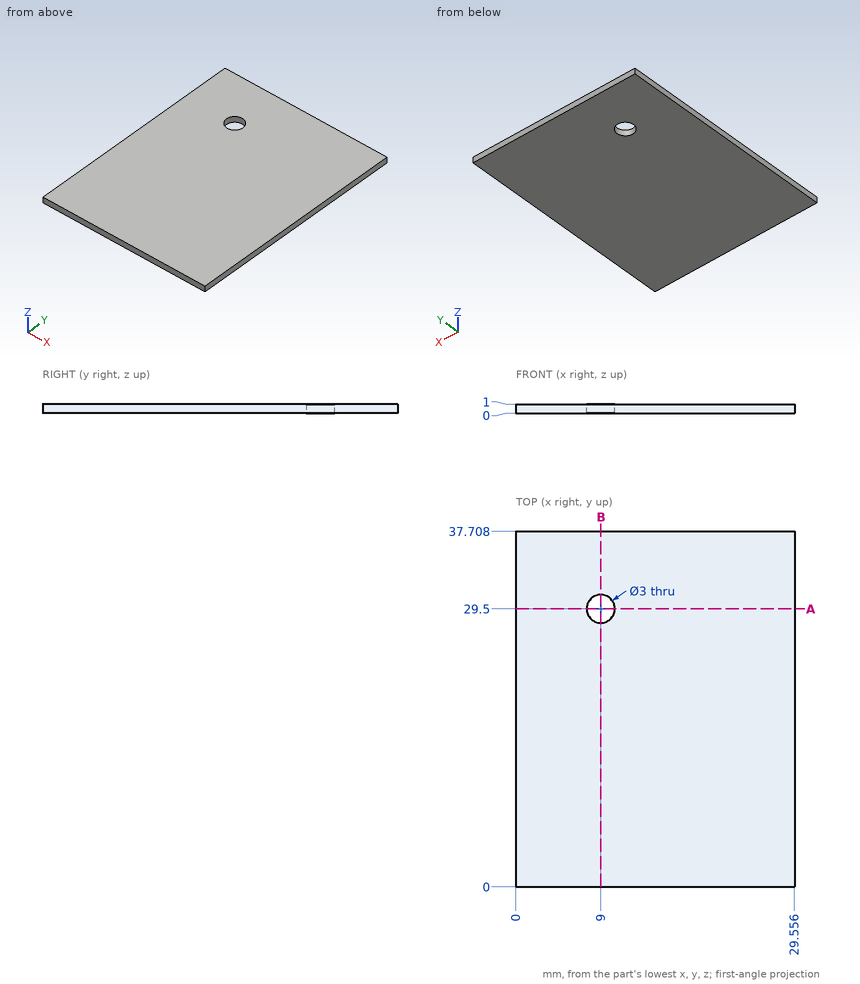
Geometry check sheet. Reference: drawing and pictorial views, mm from the part's lowest x, y, z. Round coordinates to 2 decimals unless told otherwise and drop trailing zeros. Loops run counter-clockwise (first coordinate to the right, second up) from the corner with the lowest first, then second, coordinate; pieces in that order, holes last. Notation, with made-up numbers: (25, -39) -> (59, -39) arc R10 cw to (59, -29) -> close; hole circle Ø10 at (7, 15.5). An arc over 180 degrees is marked (long way). Answer as a JSON object with one key per item and string values.
Q1. Section check A-A (y = 29.5). Record the boundary of the cut face in (x, z).
Data:
{"outline": "(0, 0) -> (7.5, 0) -> (7.5, 1) -> (0, 1) -> close; (10.5, 0) -> (29.56, 0) -> (29.56, 1) -> (10.5, 1) -> close"}
Q2. Scan lines: line 1 (X direction, y = 29.5, z = 0.35); line 2 (X direction, y = 29, z = 0.1) (1 decimal); line 3 (Y direction, x = 8, z = 0.85). Record each from-to range of solid material in increasing order. Write a range as from..to.
Data:
{"line 1": "x = 0..7.5, 10.5..29.56", "line 2": "x = 0..7.6, 10.4..29.6", "line 3": "y = 0..28.38, 30.62..37.71"}
Q3. Section check B-B (x = 9). Record the boundary of the cut face in (y, z).
Data:
{"outline": "(0, 0) -> (28, 0) -> (28, 1) -> (0, 1) -> close; (31, 0) -> (37.71, 0) -> (37.71, 1) -> (31, 1) -> close"}
